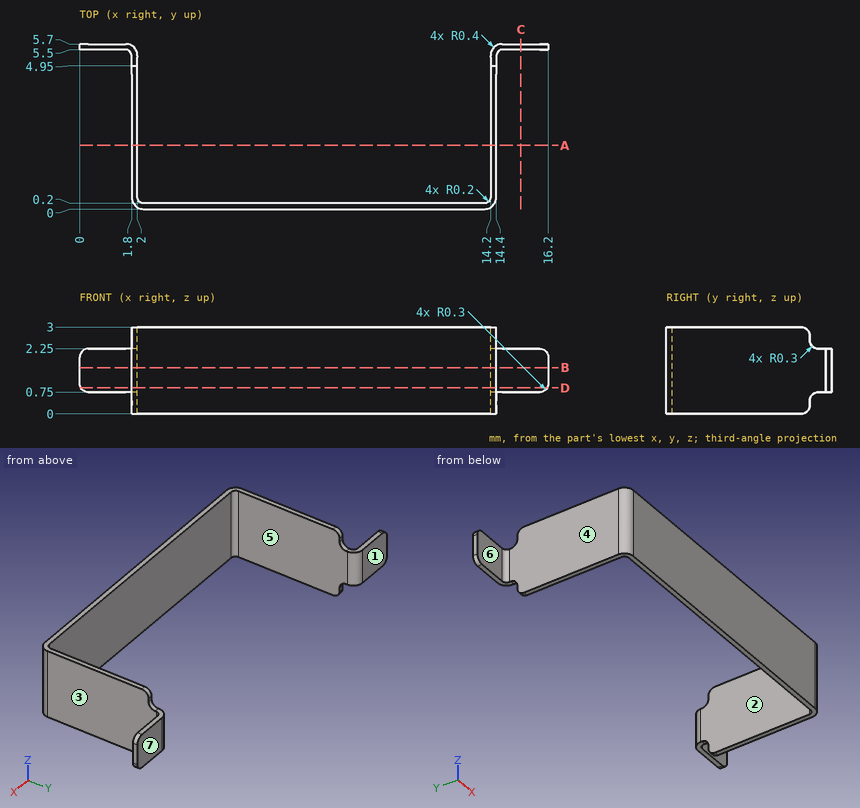
Verification items for this drawing (mm, ordinates from the low corner). A direction names the side the tool comes from. Round coordinates to 2 decimals unless told otherwise and drop trailing zeros. Loops run counter-clockwise (first coordinate to the right, second up) from the corner with the lowest first, then second, coordinate; pieces in that order, holes last. Notation, with made-up numbers: (10.25, -18) -> (44.25, -18) arc R19 ccw to (44.25, -8) -> close; hole circle Ø9 at (81, 53.5). An arc over 180 degrees is marked (long way). Answer in a Markdown table with one row per item.
Q1. Sectioned sample at C-C on x = 15.25. Enter the section's corners in (y, z).
Data:
| item | result |
|---|---|
| outline | (5.5, 0.75) -> (5.7, 0.75) -> (5.7, 2.25) -> (5.5, 2.25) -> close |
Q2. Set-up check for the marked faces 5, 6 and 7: record each of +Z, -Z, +X, -X, +Y, -Y from which the full face is reachable in a straight line by a thin tool's end or side.
Data:
| item | result |
|---|---|
| face 5 | +Z, -Z, +Y |
| face 6 | +Z, -Z, -X, -Y |
| face 7 | +Z, -Z, +X, -X, +Y |
Q3. Sectioned sample at A-A on y = 2.2. Enter the section's corners in (x, z).
Data:
| item | result |
|---|---|
| outline | (1.8, 0) -> (2, 0) -> (2, 3) -> (1.8, 3) -> close; (14.2, 0) -> (14.4, 0) -> (14.4, 3) -> (14.2, 3) -> close |
Q4. Sectioned sample at B-B on z = 1.6. Enter the section's corners in (x, y), then the cut area to 3 significant figures.
Data:
| item | result |
|---|---|
| outline | (0, 5.5) -> (1.6, 5.5) arc R0.2 cw to (1.8, 5.3) -> (1.8, 0.4) arc R0.4 ccw to (2.2, 0) -> (14, 0) arc R0.4 ccw to (14.4, 0.4) -> (14.4, 5.3) arc R0.2 cw to (14.6, 5.5) -> (16.2, 5.5) -> (16.2, 5.7) -> (14.6, 5.7) arc R0.4 ccw to (14.2, 5.3) -> (14.2, 0.4) arc R0.2 cw to (14, 0.2) -> (2.2, 0.2) arc R0.2 cw to (2, 0.4) -> (2, 5.3) arc R0.4 ccw to (1.6, 5.7) -> (0, 5.7) -> close |
| area | 5.34 mm^2 |
Q5. Sectioned sample at D-D on z = 0.9. Enter the section's corners in (x, y), then the cut area to 3 significant figures.
Data:
| item | result |
|---|---|
| outline | (0.04, 5.5) -> (1.6, 5.5) arc R0.2 cw to (1.8, 5.3) -> (1.8, 0.4) arc R0.4 ccw to (2.2, 0) -> (14, 0) arc R0.4 ccw to (14.4, 0.4) -> (14.4, 5.3) arc R0.2 cw to (14.6, 5.5) -> (16.16, 5.5) -> (16.16, 5.7) -> (14.6, 5.7) arc R0.4 ccw to (14.2, 5.3) -> (14.2, 0.4) arc R0.2 cw to (14, 0.2) -> (2.2, 0.2) arc R0.2 cw to (2, 0.4) -> (2, 5.3) arc R0.4 ccw to (1.6, 5.7) -> (0.04, 5.7) -> close |
| area | 5.32 mm^2 |
Q6. Release check for a two-part mould opening along X. For the marked faces 1, 2, 3 and 4 record: released by +X, released by -X, zero draft, split by the parting line, or undercut.
Data:
| item | result |
|---|---|
| face 1 | zero draft |
| face 2 | undercut |
| face 3 | released by +X |
| face 4 | released by -X |
Q7. Go/stop test with flat-tipped pins: P1, Ø0.9, axis at x = 7.5, z = 1.5, coming from the +Y side; P2, Ø1, axis at x = 14, z = 2, coming from the +Y side; P3, Ø1.5, axis at y = 2, z = 1.5, coming from the -X side. Record where each tip stops, or that it passes through.
Data:
| item | result |
|---|---|
| P1 | stops at y = 0.2 |
| P2 | stops at y = 5.69 |
| P3 | stops at x = 1.8 |
Q8. Thickness scan on L1, parallel to X at y = 3.55, z = 1.3; L2, parallel to Y at x = 10.75, z = 0.3. Record the ranges inside material, lowest first.
Data:
| item | result |
|---|---|
| L1 | x = 1.8 to 2, 14.2 to 14.4 |
| L2 | y = 0 to 0.2 |
